Check sheet for the modelled part. Datum: model origin and axes. Units: mm. Face numbers are marked on the shaded views. A direction names the side the tool comes from. Give positions to 0.01 mm unless a question says otherwise; leave off trailing zeros.
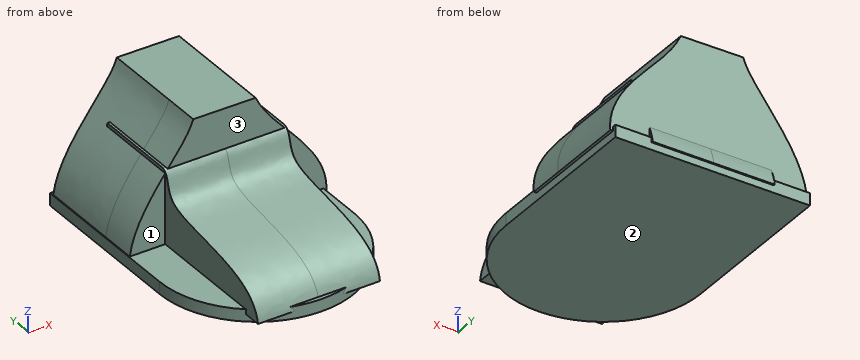
```python
from build123d import *

# Parameters (mm, degrees)
F1_DEPTH = 5.08
F3_DEPTH = 25.4
F5_DEPTH = 33.02
F6_DEPTH = 15.24


with BuildPart() as f1:
    # F0 (on Top) → F1 (new body)
    with BuildSketch(Plane.XY):
        with BuildLine():
            Line((40.5150838196, 34.5398373902), (-40.5150838196, 34.5398373902))
            Line((-40.5150838196, 34.5398373902), (-40.5150838196, -34.5398373902))
            ThreePointArc((-40.5150838196, -34.5398373902), (0, 5.9752464294), (40.5150838196, -34.5398373902))
            Line((40.5150838196, -34.5398373902), (40.5150838196, 34.5398373902))
        make_face()
        with BuildLine():
            Line((40.5150838196, -34.5398373902), (-40.5150838196, -34.5398373902))
            ThreePointArc((-40.5150838196, -34.5398373902), (0, -75.0549212098), (40.5150838196, -34.5398373902))
        make_face()
        with BuildLine():
            ThreePointArc((40.5150838196, -34.5398373902), (0, 5.9752464294), (-40.5150838196, -34.5398373902))
            Line((-40.5150838196, -34.5398373902), (40.5150838196, -34.5398373902))
        make_face()
    extrude(amount=F1_DEPTH)

    # F2 (on Right) → F3 (join, symmetric)
    with BuildSketch(Plane.YZ):
        with BuildLine():
            add(Edge.make_bspline(
                [(-73.7831778799, 3.0678272283), (-70.6378319232, 22.3217949024), (-10.9266128412, 15.6811594859), (-18.1588420727, 33.9181525964), (-13.7011114068, 35.6362367988)],
                knots=[0.0191217668, 0.0191217668, 0.0191217668, 0.0191217668, 0.4018269316, 0.5919587241, 0.5919587241, 0.5919587241, 0.5919587241], degree=3))
            Line((-73.7831778799, 3.0678272283), (35.1335004454, 3.0678272283))
            add(Edge.make_bspline(
                [(30.7071413344, 14.3951700711), (32.9333158099, 10.6251919955), (34.7726278071, 6.8872618686), (35.1335004454, 3.0678272283)],
                knots=[22.7167068517, 22.7167068517, 22.7167068517, 22.7167068517, 35.3870772104, 35.3870772104, 35.3870772104, 35.3870772104], degree=3))
            add(Edge.make_bspline(
                [(-5.1760206943, 35.6362367988), (5.8640768802, 33.5861974627), (22.7244588555, 25.6392571161), (30.7071413344, 14.3951700711)],
                knots=[0.6706583551, 0.6706583551, 0.6706583551, 0.6706583551, 0.9080645562, 0.9080645562, 0.9080645562, 0.9080645562], degree=3))
            Line((-5.1760206943, 35.6362367988), (-13.7011114068, 35.6362367988))
        make_face()
        with BuildLine():
            Line((21.2935607223, 35.6362367988), (-5.1760206943, 35.6362367988))
            add(Edge.make_bspline(
                [(-5.1760206943, 35.6362367988), (5.8640768802, 33.5861974627), (22.7244588555, 25.6392571161), (30.7071413344, 14.3951700711)],
                knots=[0.6706583551, 0.6706583551, 0.6706583551, 0.6706583551, 0.9080645562, 0.9080645562, 0.9080645562, 0.9080645562], degree=3))
            add(Edge.make_bspline(
                [(21.2935607223, 35.6362367988), (21.4809592492, 28.0165751791), (26.7158331461, 21.154363714), (30.7071413344, 14.3951700711)],
                knots=[0, 0, 0, 0, 22.7167068517, 22.7167068517, 22.7167068517, 22.7167068517], degree=3))
        make_face()
    extrude(amount=F3_DEPTH, both=True)

    # F4 (on Front) → F5 (join)
    with BuildSketch(Plane.XZ):
        with BuildLine():
            add(Edge.make_bspline(
                [(-40.2236059308, 4.5178690925), (-38.8947765504, 16.0087846112), (-25.0619320783, 34.8989974455), (-15.2672747918, 47.4251347969), (-13.7114411046, 52.3374542614)],
                knots=[0, 0, 0, 0, 0.5679803837, 1, 1, 1, 1], degree=3))
            Line((-40.2236059308, 4.5178690925), (41.6402526972, 3.2805741205))
            add(Edge.make_bspline(
                [(41.6402526972, 3.2805741205), (42.7852350273, 15.8196156508), (23.6680326777, 36.0266209863), (15.1578339465, 45.9356905739), (12.2352372609, 52.131823212)],
                knots=[0, 0, 0, 0, 0.5715646471, 1, 1, 1, 1], degree=3))
            Line((12.2352372609, 52.131823212), (-13.7114411046, 52.3374542614))
        make_face()
    extrude(amount=-F5_DEPTH)

    # F6 (add): faces of the model
    f6_faces = [f1.faces().sort_by_distance(p)[0] for p in [
        (-30.9475525695, 0, 15.5197286926),
        (-0.4224029854, 0, 43.046373164),
        (31.8842501294, 0, 15.7413854747),
    ]]
    extrude(f6_faces, amount=F6_DEPTH)


solid = f1.part
```
(1) Material ranges on line 1 (Z direction, x = -27, y = -60); line 2 (X direction, y = -64, z = 9.5); line 3 (Y direction, x = 1, z = 49), recorded low to high.
(2) Access from +Z, -Z, +X, -X, +Y, -Y to the whole of each face (thin tool, end or side, straight path). Record for the marked faces 1, 2 and 3.
(3) Gauge pin test, flat ends, axial feed: pin 1 Ø5 at (y, z) = (-21.5, 17) entering from -X; pin 2 Ø0.9 at (x, y) = (-25, -4.5) entering from +Z; pin 3 Ø12 at (x, z) = (-35.5, 13) entering from -Y. Record the tip position at first contact, or that the pin passes through.
Computed values:
1. line 1: z = 0 to 5.08
1. line 2: x = -25.4 to 25.4
1. line 3: y = -15.24 to 33.02
2. face 1: +Z, -X, -Y
2. face 2: -Z, +X, -X, +Y, -Y
2. face 3: +Z, +X, -X, -Y
3. pin 1: stops at x = -25.4
3. pin 2: stops at z = 35.64
3. pin 3: stops at y = -15.24
